```python
from build123d import *

# Parameters (mm, degrees)
FILLET1_R        = 0.2
HEX_2_DEPTH      = 1.9
EXTRUSION1_START = -0.8
ESQUISSE1_R      = 4.715
EXTRUSION1_DEPTH = 0.8


with BuildPart() as part:
    # BodySke → BaseBody (revolve)
    with BuildSketch(Plane.XY, mode=Mode.PRIVATE) as basebody_sk:
        Polygon((0, 0), (0, 4.715), (0.885, 4.715), (3.1, 2.5), (15.555, 2.5), (16, 2.055), (16, 0), align=None)
    revolve(basebody_sk.sketch.rotate(Axis((0, 0, 0), (1, 0, 0)), 90), axis=Axis((0, 0, 0), (1, 0, 0)))

    # Fillet1
    fillet1_edges = [part.edges().sort_by_distance(p)[0] for p in [
        (3.1, 0, -2.5),
    ]]
    fillet(fillet1_edges, radius=FILLET1_R)

    # Sketch2 → PreBroach (revolve, cut)
    with BuildSketch(Plane.XY, mode=Mode.PRIVATE) as prebroach_sk:
        Polygon((0, 1.5), (1.9, 1.5), (2.766025404, 0), (0, 0), align=None)
    revolve(prebroach_sk.sketch.rotate(Axis((0, 0, 0), (1, 0, 0)), 90), axis=Axis((0, 0, 0), (1, 0, 0)), mode=Mode.SUBTRACT)

    # Sketch3 → Hex 2 (cut)
    with BuildSketch(Plane.ZY):
        Polygon((-1.5, -0.866025404), (-1.5, 0.866025404), (0, 1.732050808), (1.5, 0.866025404), (1.5, -0.866025404), (0, -1.732050808), align=None)
    extrude(amount=-HEX_2_DEPTH, mode=Mode.SUBTRACT)

    # Esquisse1 → Extrusion1 (cut)
    with BuildSketch(Plane.ZY.offset(EXTRUSION1_START)):
        Circle(ESQUISSE1_R)
    extrude(amount=EXTRUSION1_DEPTH, mode=Mode.SUBTRACT)


solid = part.part
```
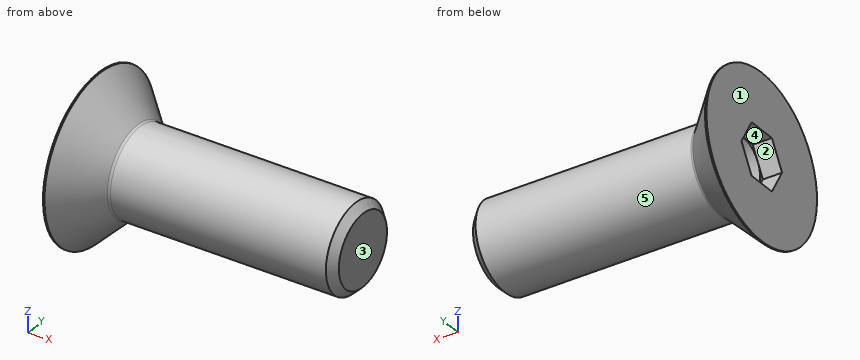
Part model, mm, in its own coordinate system. Face numbers are marked on the shaded views. A direction names the side the tool comes from. Coordinates: 2 decimals unless noted, no trailing zeros. Loops run counter-clockwise (first coordinate to the right, second up) from the corner with the lowest first, then second, coordinate; pieces in that order, holes last. Notation, with made-up numbers: (-33, -21) - (-19, -21) arc R18 cw to (-19, 2) - close; hole circle Ø4 at (78.25, 70.5). An arc over 180 degrees is marked (long way). Write item = value, one per line. Start each with the question number.
Item 1: Cut at A-A, the plane x = 11.5. Give the cut face in (y, z), and give its area (3 significant figures).
Item 2: Mould opens along Z. For the marked faces 3, 4 and 5 say: released by +Z, released by -Z, zero draft, split by the parting line, or undercut.
Item 3: Wall check: L1, parallel to Y at x = 5.75, z = 2; L2, parallel to X at y = 1.5, z = 0. Give the ranges that are in metal, low to high. Write a range as from..to.
Item 4: 3-axis set-ups, long thin cutter, end or side, ignore diameter. For the marked faces 1 and 2: which of +Z, -Z, +X, -X, +Y, -Y reach the whole face in a straight line?
Item 5: Cut at B-B, the plane x = 2.25. Give the cut face in (y, z).
Item 6: Flat gauge pins, fed straight in: pin 1 Ø5 at (x, y) = (12, 1.5) entering from -Z; pin 2 Ø0.5 at (x, y) = (1.5, 0) entering from +Z; pin 3 Ø1.5 at (x, z) = (12.5, 1.5) entering from +Y. Where does each tip first touch, or does it go through?
The answers:
q1.outline = circle Ø5 at (0, 0)
q1.area = 19.6 mm2
q2.face_3 = zero draft
q2.face_4 = undercut
q2.face_5 = split by the parting line
q3.L1 = -1.5..1.5
q3.L2 = 1.9..16
q4.face_1 = +Z, -Z, -X, +Y, -Y
q4.face_2 = -X
q5.outline = circle Ø6.7 at (0, 0); hole circle Ø1.79 at (0, 0)
q6.pin_1 = -2.5
q6.pin_2 = 4.35
q6.pin_3 = 2.38
